Here's how the part is built. I have some questions about the finished solid (model axes, mm). A direction names the side the tool comes from. Round coordinates to 2 decimals unless told otherwise and drop trailing zeros. Loops run counter-clockwise (first coordinate to the right, second up) from the corner with the lowest first, then second, coordinate; pieces in that order, holes last. Notation, with made-up numbers: (21, 0) - (30, 0) arc R21 ccw to (30, 32) - close; hole circle Ø2 at (-18, 62). An arc over 180 degrees is marked (long way). Answer as a JSON object with one key per item and string values. Group by question number.
1) I want a section at C-C, the plane y = -3.5. Please give me the cut outline in (x, z).
2) I want a section at A-A, the plane z = 0. Please give me the cut outline in (x, y), then the cut area to 3 significant figures.
3) Which directions (+Z, -Z, +X, -X, +Y, -Y) give clear straight access to the entire face, cutting with the end or side of a thin tool? Please do faces 1 (the face through (0, 72.5, 0)), 2 (the face through (-3, -64, 0)), 3 (the face through (5, 52.5, 0)), 4 (the face through (5, -52.5, 0)), 5 (the face through (-5, 52.5, 0)).
4) Will these pins go through, and if not, where does the flat tip stop? P1, Ø6, axis at x = -4.5, z = -4.5, coming from the +Y side; P2, Ø1, axis at x = 5, y = -33, coming from the -Z side; P3, Ø6, axis at y = -2.5, z = 1.5, coming from the -X side; P4, Ø4.5, axis at y = 66, z = -2, coming from the -X side.
5) If we mould it in two halves opening along Y, with no side actions, what happens to faces 6 (the face through (-0.042, 72.293, -3.082)), 7 (the face through (-0.04, -82.28, 3.12)), 8 (the face through (4.21, -0.49, 3.22))? For each: pulls with the +Y half, pulls with the -Y half, needs draft (parallel to the pull), parting line crosses it, or undercut.
6) I want a section at D-D, the plane y = 38. Please give me the cut outline in (x, z).
7) If I drill on line 1 along Y through (x, z) = (-2.25, -4.5); line 2 along Z through (x, y) = (-0.4, -75); line 3 along Y through (x, z) = (-2.5, 2), over which ranges is the centre line in solid material (lowest first)? Write a range as [from, to].
8) I want a section at B-B, the plane x = 0. Please give me the cut outline in (y, z).
from build123d import *

# Parameters (mm, degrees)
BOSS_EXTRUDE1_DEPTH     = 20
BOSS_EXTRUDE2_DEPTH     = 30
SKETCH5_R               = 5
CUT_EXTRUDE1_DEPTH      = 6
CUT_EXTRUDE1_DEPTH_BACK = 12
FILLET6_R               = 5


with BuildPart() as part:
    # Sketch1 → Revolve1 (revolve)
    with BuildSketch(Plane.XY, mode=Mode.PRIVATE) as revolve1_sk:
        with BuildLine():
            Line((0, 0), (0, -52.5))
            Line((0, -52.5), (8, -52.5))
            Line((8, -52.5), (8, -47.5))
            ThreePointArc((8, -47.5), (5.982694721, -41.39413794), (5.3, -35))
            Line((5.3, -35), (5.3, 0))
            Line((5.3, 0), (0, 0))
        make_face()
    revolve1 = revolve(revolve1_sk.sketch.rotate(Axis((0, 0, 0), (0, -1, 0)), 180), axis=Axis((0, 0, 0), (0, -1, 0)))  # turned: the seam where the file's is

    # Mirror1: Revolve1 across plane
    add(revolve1.mirror(Plane(origin=(5.3, 0, 0), x_dir=(0, 0, 1), z_dir=(0, -1, 0))))

    # Sketch3 → Boss-Extrude1 (add)
    with BuildSketch(Plane(origin=(0, 52.5, 0), x_dir=(1, 0, 0), z_dir=(0, 1, 0))):
        with BuildLine():
            Line((-3, 7.416198487), (-3, -7.416198487))
            ThreePointArc((-3, -7.416198487), (0, -8), (3, -7.416198487))
            Line((3, -7.416198487), (3, 7.416198487))
            ThreePointArc((3, 7.416198487), (0, 8), (-3, 7.416198487))
        make_face()
    extrude(amount=BOSS_EXTRUDE1_DEPTH)

    # Sketch4 → Boss-Extrude2 (add)
    with BuildSketch(Plane.XZ.offset(52.5)):
        with BuildLine():
            Line((3, 7.416198487), (3, -7.416198487))
            ThreePointArc((3, -7.416198487), (0, -8), (-3, -7.416198487))
            Line((-3, -7.416198487), (-3, 7.416198487))
            ThreePointArc((-3, 7.416198487), (0, 8), (3, 7.416198487))
        make_face()
    extrude(amount=BOSS_EXTRUDE2_DEPTH)

    # Sketch5 → Cut-Extrude1 (cut, two sides)
    with BuildSketch(Plane.ZY.offset(3)) as cut_extrude1_sk:
        with Locations(Location((0, 65, 0), (0, 0, 270))):  # turned: the seam where the file's is
            Circle(SKETCH5_R)
        with Locations(Location((0, -75, 0), (0, 0, 270))):  # turned: the seam where the file's is
            Circle(SKETCH5_R)
        with BuildLine():
            Line((-18.407176047, 86.225483422), (21.713257403, 86.225483422))
            Line((21.713257403, 86.225483422), (21.713257403, 65))
            Line((21.713257403, 65), (8, 65))
            ThreePointArc((8, 65), (0, 73), (-8, 65))
            Line((-8, 65), (-18.407176047, 65))
            Line((-18.407176047, 65), (-18.407176047, 86.225483422))
        make_face()
        with BuildLine():
            Line((21.713257403, -75), (8, -75))
            ThreePointArc((8, -75), (0, -83), (-8, -75))
            Line((-8, -75), (-18.407176047, -75))
            Line((-18.407176047, -75), (-18.407176047, -89.54271926))
            Line((-18.407176047, -89.54271926), (21.713257403, -89.54271926))
            Line((21.713257403, -89.54271926), (21.713257403, -75))
        make_face()
    extrude(amount=CUT_EXTRUDE1_DEPTH, mode=Mode.SUBTRACT)
    extrude(cut_extrude1_sk.sketch, amount=-CUT_EXTRUDE1_DEPTH_BACK, mode=Mode.SUBTRACT)

    # Fillet6
    fillet6_edges = [part.edges().sort_by_distance(p)[0] for p in [
        (0, -82.5, 2.783882181),
        (0, -82.5, -2.783882181),
        (0, 72.5, 2.783882181),
        (0, 72.5, -2.783882181),
    ]]
    fillet(fillet6_edges, radius=FILLET6_R)


solid = part.part
Outcome:
{
 "1": {"outline": "circle Ø10.6 at (0, 0)"},
 "2": {"outline": "(-8, -52.5) - (-3, -52.5) - (-3, -70) - (3, -70) - (3, -52.5) - (8, -52.5) - (8, -47.5) arc R30.29 cw to (5.3, -35) - (5.3, 35) arc R30.29 cw to (8, 47.5) - (8, 52.5) - (3, 52.5) - (3, 60) - (-3, 60) - (-3, 52.5) - (-8, 52.5) - (-8, 47.5) arc R30.29 cw to (-5.3, 35) - (-5.3, -35) arc R30.29 cw to (-8, -47.5) - close; (-3, -82.5) - (3, -82.5) - (3, -80) - (-3, -80) - close; (-3, 70) - (3, 70) - (3, 72.5) - (-3, 72.5) - close", "area": "1,390 mm^2"},
 "3": {"face 1": "+Z, -Z, +X, -X, +Y", "face 2": "+Z, -Z, -X, -Y", "face 3": "+Z, -Z, +X, +Y", "face 4": "+Z, -Z, +X, -Y", "face 5": "+Z, -Z, -X, +Y"},
 "4": {"P1": "y = 72.49", "P2": "z = -2.8", "P3": "x = -5.3", "P4": "through"},
 "5": {"face 6": "pulls with the +Y half", "face 7": "pulls with the -Y half", "face 8": "undercut"},
 "6": {"outline": "circle Ø10.9 at (0, 0)"},
 "7": {"line 1": "[-81.61, -77.18], [-72.82, 62.82], [67.18, 71.61]", "line 2": "[-7.99, -5], [5, 7.99]", "line 3": "[-82.49, -79.58], [-70.42, 60.42], [69.58, 72.49]"},
 "8": {"outline": "(-82.5, -1.66) arc R5 ccw to (-81.67, -4.42) arc R8 ccw to (-75, -8) - (-47.5, -8) arc R30.29 cw to (-35, -5.3) - (35, -5.3) arc R30.29 cw to (47.5, -8) - (65, -8) arc R8 ccw to (71.67, -4.42) arc R5 ccw to (72.5, -1.66) - (72.5, 1.66) arc R5 ccw to (71.67, 4.42) arc R8 ccw to (65, 8) - (47.5, 8) arc R30.29 cw to (35, 5.3) - (-35, 5.3) arc R30.29 cw to (-47.5, 8) - (-75, 8) arc R8 ccw to (-81.67, 4.42) arc R5 ccw to (-82.5, 1.66) - close; hole circle Ø10 at (-75, 0); hole circle Ø10 at (65, 0)"}
}
